Read the model definition and answer for the solid it produces. Units are mm, in the model's axes. A direction names the side the tool comes from. Give positions to 0.01 mm unless a question says otherwise; leave off trailing zeros. Loops run counter-clockwise (first coordinate to the right, second up) from the corner with the lowest first, then second, coordinate; pieces in that order, holes last. Notation, with made-up numbers: (-23.5, 2) - (-19.5, 2) arc R22 cw to (-19.5, 14) - close; hole circle Ø11 at (72, 64). An arc over 180 degrees is marked (long way). Use a Markdown table: item, result. Add a question column.
Item 1: A cutting plane is placed at D-D (x = -1.5). Determine the outline of the cut face in (y, z).
Item 2: Consider probe 1 along X at (y, z) = (8, 0.9); probe 2 along Y at (x, z) = (8, 1.45); probe 3 along Y at (x, z) = (-1.75, 0.8). Determine where each line is inside the solid, lowest interval first. Write a range as [from, to].
Item 3: A cutting plane is placed at C-C (x = 7). Determine the outline of the cut face in (y, z), plus the area to 4 significant figures.
Item 4: A cutting plane is placed at B-B (y = 7). Determine the outline of the cut face in (x, z), plus the area to 3 significant figures.
Item 5: Each of these flat-tipped pins is pushed along its axis until it touches: P1, Ø0.8, axis at x = -1.5, z = 0.5, coming from the -Y side; P2, Ø2, axis at x = 7.5, z = 2.5, coming from the +Y side; P3, Ø1, axis at x = 5, y = 6.5, coming from the +Z side; P4, Ø5, axis at x = -3.5, y = 7, coming from the +Z side. Where does it stop, or does it pass through?
Item 6: For a pull along X with two mould halves and no side action, classify faces 1 (the face through (-8, -16, 4.5)), 2 (the face through (8.75, -6.2, 0.6)), 3 (the face through (-6.25, -7.2, 0.6)) as +X half, -X half, draft (parallel to the pull), parting line (faces both ways), or undercut.
Item 7: A cutting plane is placed at A-A (z = 4). Determine the outline of the cut face in (x, y).
Item 8: Which of the six approach directions +Z, -Z, +X, -X, +Y, -Y give full straight-line access (tool end or side, diameter ignored) to faces 4 (the face through (7, -16, 4.5)), 5 (the face through (-0.1, 8.75, 0.5)), 6 (the face through (-8, -14.75, 3))?
from build123d import *

# Parameters (mm, degrees)
SKETCH1_W           = 2.5
SKETCH1_H           = 26
BOSS_EXTRUDE1_DEPTH = 1
SKETCH2_W           = 2.5
SKETCH2_H           = 2.5
BOSS_EXTRUDE2_DEPTH = 3.5


with BuildPart() as part:
    # Sketch1 → Boss-Extrude1 (new body)
    with BuildSketch(Plane.XY):
        with Locations((-7.5, -4.25)):
            Rectangle(SKETCH1_W, SKETCH1_H)
        Polygon((-8.75, 11.25), (-8.75, 8.75), (-6.25, 8.75), (6.25, 8.75), (8.75, 8.75), (8.75, 11.25), align=None)
        with Locations((7.5, -4.25)):
            Rectangle(SKETCH1_W, SKETCH1_H)
    extrude(amount=BOSS_EXTRUDE1_DEPTH)

    # Sketch2 → Boss-Extrude2 (add)
    with BuildSketch(Plane.XY.offset(1)):
        with Locations((-7.5, -16)):
            Rectangle(SKETCH2_W, SKETCH2_H)
        with Locations((7.5, -16)):
            Rectangle(SKETCH2_W, SKETCH2_H)
    extrude(amount=BOSS_EXTRUDE2_DEPTH)


solid = part.part
Geometry says:
| question | item | result |
|---|---|---|
| 1 | outline | (8.75, 0) - (11.25, 0) - (11.25, 1) - (8.75, 1) - close |
| 2 | probe 1 | [-8.75, -6.25], [6.25, 8.75] |
| 2 | probe 2 | [-17.25, -14.75] |
| 2 | probe 3 | [8.75, 11.25] |
| 3 | outline | (-17.25, 0) - (11.25, 0) - (11.25, 1) - (-14.75, 1) - (-14.75, 4.5) - (-17.25, 4.5) - close |
| 3 | area | 37.25 mm² |
| 4 | outline | (-8.75, 0) - (-6.25, 0) - (-6.25, 1) - (-8.75, 1) - close; (6.25, 0) - (8.75, 0) - (8.75, 1) - (6.25, 1) - close |
| 4 | area | 5.00 mm² |
| 5 | P1 | y = 8.75 |
| 5 | P2 | y = -14.75 |
| 5 | P3 | through |
| 5 | P4 | z = 1 |
| 6 | face 1 | draft |
| 6 | face 2 | +X half |
| 6 | face 3 | undercut |
| 7 | outline | (-8.75, -17.25) - (-6.25, -17.25) - (-6.25, -14.75) - (-8.75, -14.75) - close; (6.25, -17.25) - (8.75, -17.25) - (8.75, -14.75) - (6.25, -14.75) - close |
| 8 | face 4 | +Z, +X, -X, +Y, -Y |
| 8 | face 5 | +Z, -Z, -Y |
| 8 | face 6 | +Z, +X, -X, +Y |
